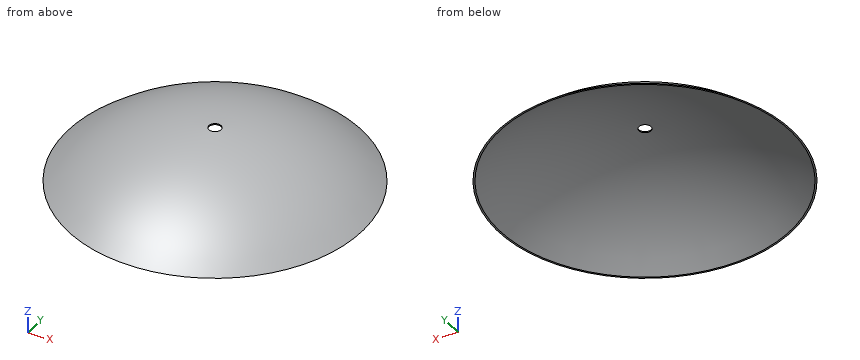
```python
from build123d import *

# Parameters (mm, degrees)
F3_T     = -1
F2_R     = 5.5
F4_DEPTH = 25.001


with BuildPart() as f1:
    # F0 (on Front) → F1 (revolve)
    with BuildSketch(Plane.XZ):
        with BuildLine():
            Line((0, 25), (0, -25))
            Line((0, -25), (133, -25))
            ThreePointArc((133, -25), (71.0440004504, 12.0870411981), (0, 25))
        make_face()
    revolve(axis=Axis((0, 0, 0), (0, 0, -1)))

    # F3
    f3_openings = [f1.faces().sort_by_distance(p)[0] for p in [
        (0, 0, -25),
    ]]
    offset(amount=F3_T, openings=f3_openings)

    # F2 (on Top) → F4 (cut, through all)
    with BuildSketch(Plane.XY):
        Circle(F2_R)
    extrude(amount=F4_DEPTH, mode=Mode.SUBTRACT)


solid = f1.part
```
Can you work these out from the model? Positions are in its coordinate system, mm. Coordinates: 2 decimals unless noted, no trailing zeros. Loops run counter-clockwise (first coordinate to the right, second up) from the corner with the lowest first, then second, coordinate; pieces in that order, holes last.
1) For pin 1 (1 mm diameter, centred on x = 99.5, y = 15, fed in from -Z); pin 2 (12 mm diameter, centred on x = 13, z = -15.5, fed in from +Y); pin 3 (1.5 mm diameter, centred on x = -3, z = -8.5, fed in from -Y), each with a flat end and sliding along its axis, tell me the tip position at first contact or that it passes through.
2) Imagine slicing it at A-A on y = 0. List the corners of the cut face in (x, z) for me.
3) I need wall thicknesses on probe 1 along X at (y, z) = (17, -4.5); probe 2 along X at (y, z) = (12, -10); probe 3 along Y at (x, z) = (53, -3). Which ranges of each line are inside material? Lowest first, please.
4) Imagine slicing it at D-D on y = 29. List the corners of the cut face in (x, z) for me, plus the area to 3 significant figures.
Completed:
1. pin 1: stops at z = -3.31
1. pin 2: stops at y = 128.26
1. pin 3: stops at y = -112.46
2. outline: (-133, -25) - (-131.48, -25) arc R200.89 cw to (-5.5, 23.92) - (-5.5, 24.93) arc R201.89 ccw to start; (5.5, 23.92) arc R200.89 cw to (131.48, -25) - (133, -25) arc R201.89 ccw to (5.5, 24.93) - close
3. probe 1: x = -103.69 to -101.73, 101.73 to 103.69
3. probe 2: x = -112.97 to -111.18, 111.18 to 112.97
3. probe 3: y = -87.82 to -85.5, 85.5 to 87.82
4. outline: (-129.8, -25) - (-128.24, -25) arc R198.79 cw to (128.24, -25) - (129.8, -25) arc R199.8 ccw to start
4. area: 284 mm2
